```python
from build123d import *

# Parameters (mm, degrees)
SKETCH1_W                   = 12.7
SKETCH1_H                   = 12.7
BOSS_EXTRUDE1_DEPTH         = 2.54
M3_CLEARANCE_HOLE1_D        = 3.4
TAP_DRILL_FOR_M3X0_5_TAP1_D = 2.5


with BuildPart() as part:
    # Sketch1 → Boss-Extrude1 (new body)
    with BuildSketch(Plane(origin=(0, 0, 0), x_dir=(1, 0, 0), z_dir=(0, 1, 0))):
        Rectangle(SKETCH1_W, SKETCH1_H)
    extrude(amount=BOSS_EXTRUDE1_DEPTH)

    # M3 Clearance Hole1 (through all)
    with Locations(Plane(origin=(0, 2.54, -2.54), x_dir=(0, 0, 1), z_dir=(0, 1, 0))):
        with Locations((0, 0)):
            Hole(M3_CLEARANCE_HOLE1_D / 2)

    # Tap Drill for M3x0.5 Tap1 (through all)
    with Locations(Plane(origin=(0, 2.54, 2.54), x_dir=(0, 0, 1), z_dir=(0, 1, 0))):
        with Locations((0, 0)):
            Hole(TAP_DRILL_FOR_M3X0_5_TAP1_D / 2)


solid = part.part
```
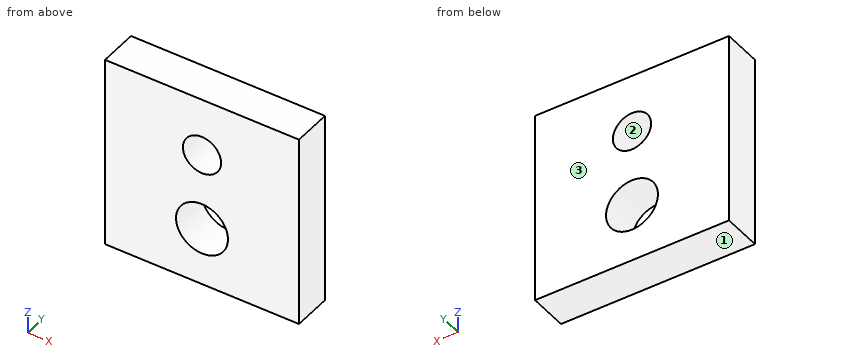
Check sheet for the modelled part. Datum: model origin and axes. Units: mm. Face numbers are marked on the shaded views. Round coordinates to 2 decimals unless told otherwise and drop trailing zeros. Write each loop counter-clockwise with the first axis right and the second up, starting at its lowest first coordinate (ties: lowest second). Pieces come first, ordered by that corner, then holes. Notation, with made-up numbers: (48.5, -15) -> (105.5, -15) arc R15 cw to (105.5, 7) -> close; hole circle Ø7 at (16.5, -30). An arc over 180 degrees is marked (long way). One line per question, with ' | ' between items. Start each with the question number.
1. Sectioned sample at B-B, the plane z = 2.54. Record the cut outline in (x, y), then the cut area to 3 significant figures.
2. Sectioned sample at C-C, the plane y = 0.65. Record the cut outline in (x, z), then the cut area to 3 significant figures.
3. Release check for a two-part mould opening along Z. For the marked faces 1, 2 and 3 record: +Z half, -Z half, draft (parallel to the pull), parting line (faces both ways), or undercut.
4. Sectioned sample at A-A, the plane x = 0. Record the cut outline in (y, z).
5. Scan lines: line 1 along X through (y, z) = (0.95, -2.54); line 2 along X through (y, z) = (0.9, 2.54); line 3 along Z through (x, y) = (1, 0.85). Record each from-to range of solid material in increasing order. Write a range as from..to.
6. Sectioned sample at D-D, the plane z = -2.54. Record the cut outline in (x, y).
Taken from the geometry:
1) outline: (-6.35, 0) -> (-1.25, 0) -> (-1.25, 2.54) -> (-6.35, 2.54) -> close; (1.25, 0) -> (6.35, 0) -> (6.35, 2.54) -> (1.25, 2.54) -> close | area: 25.9 mm^2
2) outline: (-6.35, -6.35) -> (6.35, -6.35) -> (6.35, 6.35) -> (-6.35, 6.35) -> close; hole circle Ø3.4 at (0, -2.54); hole circle Ø2.5 at (0, 2.54) | area: 147 mm^2
3) face 1: -Z half | face 2: undercut | face 3: draft
4) outline: (0, -6.35) -> (2.54, -6.35) -> (2.54, -4.24) -> (0, -4.24) -> close; (0, -0.84) -> (2.54, -0.84) -> (2.54, 1.29) -> (0, 1.29) -> close; (0, 3.79) -> (2.54, 3.79) -> (2.54, 6.35) -> (0, 6.35) -> close
5) line 1: x = -6.35..-1.7, 1.7..6.35 | line 2: x = -6.35..-1.25, 1.25..6.35 | line 3: z = -6.35..-3.91, -1.17..1.79, 3.29..6.35
6) outline: (-6.35, 0) -> (-1.7, 0) -> (-1.7, 2.54) -> (-6.35, 2.54) -> close; (1.7, 0) -> (6.35, 0) -> (6.35, 2.54) -> (1.7, 2.54) -> close
